from build123d import *

# Parameters (mm, degrees)
SKETCH_1_R           = 8
EXTRUDE_2_DEPTH      = 2
EXTRUDE_3_DEPTH      = 18
EXTRUDE_3_DEPTH_BACK = 1
SKETCH_2_W           = 45.2
SKETCH_2_H           = 2
SKETCH_3_W           = 45.2
SKETCH_3_H           = 18
EXTRUDE_4_DEPTH      = 18
SKETCH_4_W           = 45.2
SKETCH_4_H           = 18
CUT_EXTRUDE_2_DEPTH  = 16
CUT_EXTRUDE_4_DEPTH  = 20
SKETCH_7_W           = 0.117046
SKETCH_7_H           = 18
CUT_EXTRUDE_5_DEPTH  = 20
CUT_EXTRUDE_6_DEPTH  = 20
SKETCH_9_R           = 0.5
CUT_EXTRUDE_7_DEPTH  = 20
CUT_EXTRUDE_8_DEPTH  = 20
FILLET_1_R           = 1
FILLET_2_R           = 1
FILLET_3_R           = 1
SKETCH_14_W          = 47.954779
SKETCH_14_H          = 7.292093
CUT_EXTRUDE_12_DEPTH = 4
EXTRUDE_START        = -4
EXTRUDE_11_OUTLINE_R = 8
EXTRUDE_11_DEPTH     = 4


# Read off the part's stored shape, not the designer's step: 凸台-拉伸11
with BuildPart() as part:
    # 草图1 → 凸台-拉伸2 (new body)
    with BuildSketch(Plane.XY):
        with BuildLine():
            Line((1, 0), (44.2, 0))
            ThreePointArc((44.2, 0), (44.907107, 0.292893), (45.2, 1))
            Line((45.2, 1), (45.2, 19.33))
            ThreePointArc((45.2, 19.33), (44.907107, 20.037107), (44.2, 20.33))
            Line((44.2, 20.33), (1, 20.33))
            ThreePointArc((1, 20.33), (0.292893, 20.037107), (0, 19.33))
            Line((0, 19.33), (0, 1))
            ThreePointArc((0, 1), (0.292893, 0.292893), (1, 0))
        make_face()
        with Locations((35.6, 10.165)):
            Circle(SKETCH_1_R, mode=Mode.SUBTRACT)
        with Locations((9.6, 10.165)):
            Circle(SKETCH_1_R, mode=Mode.SUBTRACT)
    extrude(amount=EXTRUDE_2_DEPTH)

    # 草图2 → 凸台-拉伸3 (add, two sides: drawn at the far end of the back side and taken through both)
    with BuildSketch(Plane.XZ.offset(-EXTRUDE_3_DEPTH_BACK)):
        with Locations((22.6, 1)):
            Rectangle(SKETCH_2_W, SKETCH_2_H)
    extrude(amount=EXTRUDE_3_DEPTH + EXTRUDE_3_DEPTH_BACK)

    # 草图3 → 凸台-拉伸4 (add)
    with BuildSketch(Plane(origin=(0, 0, 0), x_dir=(-1, 0, 0), z_dir=(0, 0, -1))):
        with Locations((-22.6, -9)):
            Rectangle(SKETCH_3_W, SKETCH_3_H)
    extrude(amount=EXTRUDE_4_DEPTH)

    # 草图4 → 切除-拉伸2 (cut)
    with BuildSketch(Plane(origin=(0, 0, 0), x_dir=(1, 0, 0), z_dir=(0, 1, 0))):
        with Locations((22.6, 9)):
            Rectangle(SKETCH_4_W, SKETCH_4_H)
    extrude(amount=-CUT_EXTRUDE_2_DEPTH, mode=Mode.SUBTRACT)

    # 草图5 → 切除-拉伸4 (cut)
    with BuildSketch(Plane.XY.offset(2)):
        Polygon((0, -18), (5.6, -18), (0, -2), align=None)
        with BuildLine():
            Line((0, -2), (5.6, -18))
            add(Edge.make_bspline(
                [(0, -2), (5.393134, -9.559308), (5.6, -18)],
                knots=[0, 0, 0, 0.926119, 0.926119, 0.926119], degree=2))
        make_face()
        with BuildLine():
            add(Edge.make_bspline(
                [(45.2, -2), (39.778817, -9.554541), (39.6, -18)],
                knots=[0, 0, 0, 0.936137, 0.936137, 0.936137], degree=2))
            Line((39.6, -18), (45.2, -18))
            Line((45.2, -18), (45.2, -2))
        make_face()
    extrude(amount=-CUT_EXTRUDE_4_DEPTH, mode=Mode.SUBTRACT)

    # 草图7 → 切除-拉伸5 (cut)
    with BuildSketch(Plane(origin=(0, -18, 0), x_dir=(-1, 0, 0), z_dir=(0, -1, 0))):
        with Locations((-39.658523, 9)):
            Rectangle(SKETCH_7_W, SKETCH_7_H)
    extrude(amount=-CUT_EXTRUDE_5_DEPTH, mode=Mode.SUBTRACT)

    # 草图8 → 切除-拉伸6 (cut)
    with BuildSketch(Plane(origin=(0, -18, 0), x_dir=(-1, 0, 0), z_dir=(0, -1, 0))):
        with BuildLine():
            ThreePointArc((-39.6, 17), (-39.307107, 17.707107), (-38.6, 18))
            Line((-38.6, 18), (-39.6, 18))
            Line((-39.6, 18), (-39.6, 17))
        make_face()
        with BuildLine():
            ThreePointArc((-6.6, 18), (-5.892893, 17.707107), (-5.6, 17))
            Line((-5.6, 17), (-5.6, 18))
            Line((-5.6, 18), (-6.6, 18))
        make_face()
        Polygon((-5.6, 0), (-5.476967, 0), (-5.476967, 18), (-5.6, 18), (-5.6, 17), align=None)
    extrude(amount=-CUT_EXTRUDE_6_DEPTH, mode=Mode.SUBTRACT)

    # 草图9 → 切除-拉伸7 (cut)
    with BuildSketch(Plane.XZ.offset(18)):
        with Locations(Location((16.35, -9, 0), (0, 0, 270))):
            Circle(SKETCH_9_R)
        with Locations(Location((22.6, -2.75, 0), (0, 0, 270))):
            Circle(SKETCH_9_R)
        with Locations(Location((28.85, -9, 0), (0, 0, 270))):
            Circle(SKETCH_9_R)
        with Locations(Location((22.6, -15.25, 0), (0, 0, 270))):
            Circle(SKETCH_9_R)
    extrude(amount=-CUT_EXTRUDE_7_DEPTH, mode=Mode.SUBTRACT)

    # 草图10 → 切除-拉伸8 (cut)
    with BuildSketch(Plane.XY.offset(2)):
        Polygon((22.6, 20.33), (17.1, 20.33), (17.1, 14.83), (28.1, 14.83), (28.1, 20.33), align=None)
    extrude(amount=-CUT_EXTRUDE_8_DEPTH, mode=Mode.SUBTRACT)

    # 圆角1
    fillet_1_edges = [part.edges().sort_by_distance(p)[0] for p in [
        (28.1, 20.33, 1),
        (17.1, 20.33, 1),
    ]]
    fillet(fillet_1_edges, radius=FILLET_1_R)

    # 圆角2
    fillet_2_edges = [part.edges().sort_by_distance(p)[0] for p in [
        (28.1, 14.83, 1),
    ]]
    fillet(fillet_2_edges, radius=FILLET_2_R)

    # 圆角3
    fillet_3_edges = [part.edges().sort_by_distance(p)[0] for p in [
        (17.1, 14.83, 1),
    ]]
    fillet(fillet_3_edges, radius=FILLET_3_R)

    # 草图14 → 切除-拉伸12 (cut)
    with BuildSketch(Plane(origin=(0, 20.33, 0), x_dir=(1, 0, 0), z_dir=(0, 1, 0))):
        with Locations((22.880684, -2.280867)):
            Rectangle(SKETCH_14_W, SKETCH_14_H)
    extrude(amount=-CUT_EXTRUDE_12_DEPTH, mode=Mode.SUBTRACT)

    # 凸台-拉伸11 outline → 凸台-拉伸11 (add)
    with BuildSketch(Plane.XY.offset(2).offset(EXTRUDE_START)):
        with BuildLine():
            add(Edge.make_bspline(
                [(0, -2), (5.393134, -9.559308), (5.6, -18)],
                knots=[0, 0, 0, 0.926119, 0.926119, 0.926119], degree=2))
            Line((5.6, -18), (5.6, -16))
            Line((5.6, -16), (39.6, -16))
            Line((39.6, -16), (39.6, -18))
            add(Edge.make_bspline(
                [(45.2, -2), (39.778817, -9.554541), (39.6, -18)],
                knots=[0, 0, 0, 0.936137, 0.936137, 0.936137], degree=2))
            Line((45.2, -2), (45.2, 16.83))
            add(Edge.make_bspline(
                [(36.65, 26.38), (41.993745, 20.411254), (44.982894, 20.749172), (45.2, 16.83)],
                knots=[0, 0, 0, 0, 0.927631, 0.927631, 0.927631, 0.927631], degree=3))
            add(Edge.make_bspline(
                [(36.65, 26.38), (31.306253, 20.41125), (28.317106, 20.749171), (28.1, 16.83)],
                knots=[0, 0, 0, 0, 0.927631, 0.927631, 0.927631, 0.927631], degree=3))
            Line((28.1, 16.83), (28.1, 15.83))
            ThreePointArc((28.1, 15.83), (27.807107, 15.122893), (27.1, 14.83))
            Line((27.1, 14.83), (18.1, 14.83))
            ThreePointArc((18.1, 14.83), (17.392893, 15.122893), (17.1, 15.83))
            Line((17.1, 15.83), (17.1, 16.83))
            add(Edge.make_bspline(
                [(8.55, 26.38), (13.893745, 20.411254), (16.882894, 20.749172), (17.1, 16.83)],
                knots=[0, 0, 0, 0, 0.927631, 0.927631, 0.927631, 0.927631], degree=3))
            add(Edge.make_bspline(
                [(8.55, 26.38), (3.206253, 20.41125), (0.217106, 20.749171), (0, 16.83)],
                knots=[0, 0, 0, 0, 0.927631, 0.927631, 0.927631, 0.927631], degree=3))
            Line((0, 16.83), (0, -2))
        make_face()
        with Locations((9.6, 10.165)):
            Circle(EXTRUDE_11_OUTLINE_R, mode=Mode.SUBTRACT)
        with Locations((35.6, 10.165)):
            Circle(EXTRUDE_11_OUTLINE_R, mode=Mode.SUBTRACT)
    extrude(amount=EXTRUDE_11_DEPTH)


solid = part.part
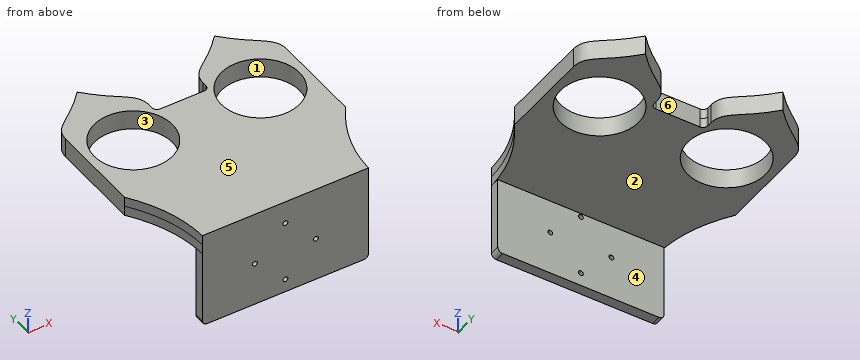
Geometry: final body of the model. Coordinates: model frame, mm. Face numbers are marked on the shaded views. A direction names the side the tool comes from. Coordinates: 2 decimals unless noted, no trailing zeros. Order: outer loops, then holes, each group sorted by start corner. A loop starts at its lowest first (then second) coordinate and runs counter-clockwise, first axis right, second up.
(1) Section query B-B (x = 26.5). Return the cut outline in (y, z).
(2) Material intervals for probe 1 along X at (y, z) = (-16.75, -9); probe 2 along X at (y, z) = (-17, -2.75); probe 3 along Z at (x, y) = (32.5, -3), sorted ascending.
(3) Section query A-A (z = -12.25). Return the cut outline in (x, y), plus the area to 3 significant figures.
(4) Access query for the marked faces 4, 5 and 6. Directions: +Z, -Z, +X, -X, +Y, -Y. A direction counts if a zero-diameter tool reaches every point of the face in a straight line with its end or side. Return the directions, or none.
(5) First-contact query: pin 1 (9.5 mm diameter, centred on x = 9.6, y = 10.165, fed in from -Z); pin 2 (2 mm diameter, centred on y = -17.5, z = -6, fed in from -X); pin 3 (0.6 mm diameter, centred on y = -16.5, z = -6, fed in from +X); pin 4 (6 mm diameter, centred on x = 34.5, z = -8.5, fed in from +Y). Flat tips, straight axial feed; report the tip coordinate or a pass-through.
(6) Draft query along X for the marked faces 1, 2 and 3. Return one class per face: pulls with the +X half, pulls with the -X half, needs draft (parallel to the pull), parting line crosses it, or undercut.
Solution:
1. outline: (-18, -18) - (-16, -18) - (-16, -2) - (14.83, -2) - (14.83, 2) - (-18, 2) - close
2. probe 1: x = 5.6 to 15.85, 16.85 to 28.35, 29.35 to 39.6
2. probe 2: x = 5.6 to 22.1, 23.1 to 39.6
2. probe 3: z = -2 to 2
3. outline: (5.6, -18) - (39.6, -18) - (39.6, -16) - (5.6, -16) - close
3. area: 68.0 mm2
4. face 4: -Z, +X, -X, +Y
4. face 5: +Z, +X, -X, +Y, -Y
4. face 6: +Z, -Z, +Y
5. pin 1: passes through
5. pin 2: stops at x = 5.6
5. pin 3: stops at x = 39.6
5. pin 4: stops at y = -16
6. face 1: undercut
6. face 2: needs draft
6. face 3: undercut
